Verification items for the finished model (mm, model axes). Coordinates: 2 decimals unless noted, no trailing zeros. Order: outer loops, then holes, each group sorted by start corner. A loop starts at its lowest first (then second) coordinate and runs counter-clockwise, first axis right, second up. Notation, with made-up numbers: M 76.5,-21 L 94.5,-21 A17 ccw 94.5,9 Z; hole C 20.5,43.5 d10. An arc over 180 degrees is marked long. Return JSON: item names as keys, results as strings. Group by question number.
1. Section check B-B, the plane x = 1.25. Record the cut outline in (y, z).
2. Section check C-C, the plane y = -15.5. Record the cut outline in (x, z), plus the area to 3 significant figures.
3. Section check A-A, the plane y = 0. Record the cut outline in (x, z).
4. Section check D-D, the plane x = -14.25. Record the cut outline in (y, z), plus the area to 3 significant figures.
5. Material ranges on line 1 along Y through (x, z) = (16.75, 0.4); line 2 along Y through (x, z) = (18, 1.5); line 3 along Y through (x, z) = (23.5, 1.5), recorded low to high.
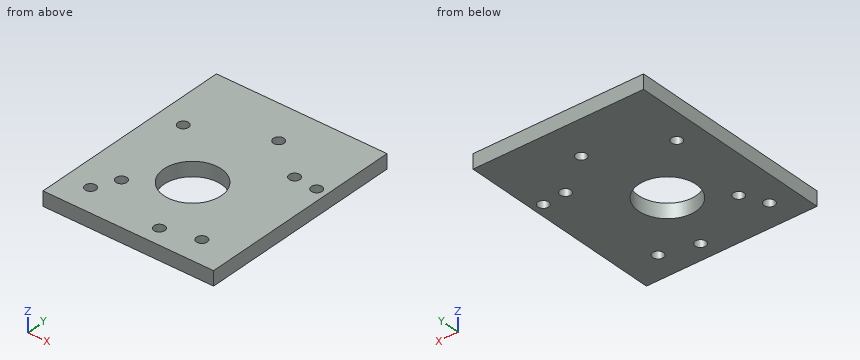
```python
from build123d import *

# Parameters (mm, degrees)
SKETCH1_W           = 42.5
SKETCH1_H           = 40
BOSS_EXTRUDE1_DEPTH = 2
SKETCH2_R           = 1.5
CUT_EXTRUDE1_DEPTH  = 4
SKETCH3_R           = 8
CUT_EXTRUDE2_DEPTH  = 4
SKETCH4_W           = 42.5
SKETCH4_H           = 4
BOSS_EXTRUDE2_DEPTH = 15
SKETCH8_W           = 4
SKETCH8_H           = 55
BOSS_EXTRUDE3_DEPTH = 5
SKETCH7_R           = 1.5
CUT_EXTRUDE3_DEPTH  = 10
SKETCH9_W           = 47.5
SKETCH9_H           = 4
BOSS_EXTRUDE4_DEPTH = 3


with BuildPart() as part:
    # Sketch1 → Boss-Extrude1 (new, symmetric)
    with BuildSketch(Plane.XY):
        Rectangle(SKETCH1_W, SKETCH1_H)
    extrude(amount=BOSS_EXTRUDE1_DEPTH, both=True)

    # Sketch2 → Cut-Extrude1 (cut)
    with BuildSketch(Plane(origin=(0, 0, -2), x_dir=(-1, 0, 0), z_dir=(0, 0, -1))):
        with Locations((-16.75, 15.5)):
            Circle(SKETCH2_R)
        with Locations((14.25, 15.5)):
            Circle(SKETCH2_R)
        with Locations((14.25, -15.5)):
            Circle(SKETCH2_R)
        with Locations((-16.75, -15.5)):
            Circle(SKETCH2_R)
    extrude(amount=-CUT_EXTRUDE1_DEPTH, mode=Mode.SUBTRACT)

    # Sketch3 → Cut-Extrude2 (cut)
    with BuildSketch(Plane.XY.offset(2)):
        with Locations((1.25, 0)):
            Circle(SKETCH3_R)
    extrude(amount=-CUT_EXTRUDE2_DEPTH, mode=Mode.SUBTRACT)

    # Sketch4 → Boss-Extrude2 (add)
    with BuildSketch(Plane(origin=(0, 20, 0), x_dir=(1, 0, 0), z_dir=(0, 1, 0))):
        Rectangle(SKETCH4_W, SKETCH4_H)
    extrude(amount=BOSS_EXTRUDE2_DEPTH)

    # Sketch8 → Boss-Extrude3 (add)
    with BuildSketch(Plane(origin=(21.25, 0, 0), x_dir=(0, 0, -1), z_dir=(1, 0, 0))):
        with Locations((0, 7.5)):
            Rectangle(SKETCH8_W, SKETCH8_H)
    extrude(amount=BOSS_EXTRUDE3_DEPTH)

    # Sketch7 → Cut-Extrude3 (cut)
    with BuildSketch(Plane.XY.offset(2)):
        with Locations((5.303802982, 23.945501151)):
            Circle(SKETCH7_R)
        with Locations((23.303478189, 15.039308246)):
            Circle(SKETCH7_R)
        with Locations((6.975457864, -17.9600963)):
            Circle(SKETCH7_R)
        with Locations((-11.024217343, -9.053903396)):
            Circle(SKETCH7_R)
    extrude(amount=-CUT_EXTRUDE3_DEPTH, mode=Mode.SUBTRACT)

    # Sketch9 → Boss-Extrude4 (add)
    with BuildSketch(Plane.XZ.offset(20)):
        with Locations((2.5, 0)):
            Rectangle(SKETCH9_W, SKETCH9_H)
    extrude(amount=BOSS_EXTRUDE4_DEPTH)


solid = part.part
```
Answers follow:
{
 "1": {"outline": "M -23,-2 L -8,-2 L -8,2 L -23,2 Z; M 8,-2 L 35,-2 L 35,2 L 8,2 Z"},
 "2": {"outline": "M -21.25,-2 L -15.75,-2 L -15.75,2 L -21.25,2 Z; M -12.75,-2 L 15.25,-2 L 15.25,2 L -12.75,2 Z; M 18.25,-2 L 26.25,-2 L 26.25,2 L 18.25,2 Z", "area": "166 mm^2"},
 "3": {"outline": "M -21.25,-2 L -6.75,-2 L -6.75,2 L -21.25,2 Z; M 9.25,-2 L 26.25,-2 L 26.25,2 L 9.25,2 Z"},
 "4": {"outline": "M -23,-2 L -17,-2 L -17,2 L -23,2 Z; M -14,-2 L 14,-2 L 14,2 L -14,2 Z; M 17,-2 L 35,-2 L 35,2 L 17,2 Z", "area": "208 mm^2"},
 "5": {"line 1": "-23 to -17, -14 to 14, 17 to 35", "line 2": "-23 to -16.33, -14.67 to 14.67, 16.33 to 35", "line 3": "-23 to 13.55, 16.53 to 35"}
}
